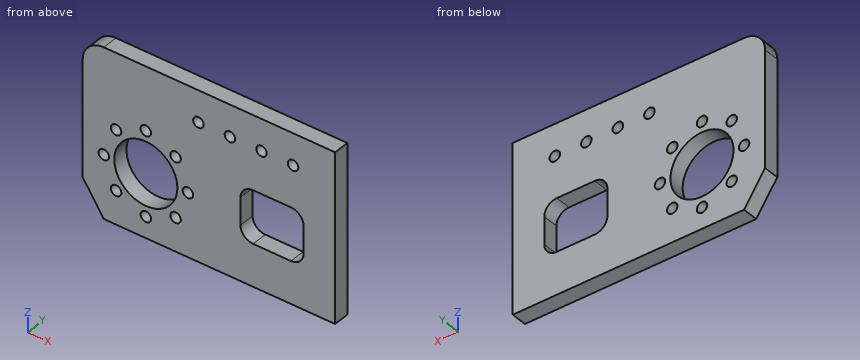
from build123d import *

# Parameters (mm, degrees)
SKETCH1_R           = 19.05
SKETCH1_R_2         = 3.175
BOSS_EXTRUDE1_DEPTH = 9.525


with BuildPart() as part:
    # Sketch1 → Boss-Extrude1 (new body)
    with BuildSketch(Plane(origin=(0, 0, 0), x_dir=(1, 0, 0), z_dir=(0, 1, 0))):
        with BuildLine():
            Line((0, -19.05), (12.7, 0))
            Line((12.7, 0), (152.4, 0))
            Line((152.4, 0), (152.4, -101.6))
            Line((152.4, -101.6), (12.7, -101.6))
            ThreePointArc((12.7, -101.6), (3.719743879, -97.880256121), (0, -88.9))
            Line((0, -88.9), (0, -19.05))
        make_face()
        with Locations((38.1, -38.1)):
            Circle(SKETCH1_R, mode=Mode.SUBTRACT)
        with Locations((56.060512242, -56.060512242)):
            Circle(SKETCH1_R_2, mode=Mode.SUBTRACT)
        with Locations((38.1, -63.5)):
            Circle(SKETCH1_R_2, mode=Mode.SUBTRACT)
        with Locations((20.139487758, -56.060512242)):
            Circle(SKETCH1_R_2, mode=Mode.SUBTRACT)
        with Locations((12.7, -38.1)):
            Circle(SKETCH1_R_2, mode=Mode.SUBTRACT)
        with Locations((20.139487758, -20.139487758)):
            Circle(SKETCH1_R_2, mode=Mode.SUBTRACT)
        with Locations((38.1, -12.7)):
            Circle(SKETCH1_R_2, mode=Mode.SUBTRACT)
        with Locations((56.060512242, -20.139487758)):
            Circle(SKETCH1_R_2, mode=Mode.SUBTRACT)
        with Locations((63.5, -38.1)):
            Circle(SKETCH1_R_2, mode=Mode.SUBTRACT)
        with Locations((69.85, -82.55)):
            Circle(SKETCH1_R_2, mode=Mode.SUBTRACT)
        with Locations((88.9, -82.55)):
            Circle(SKETCH1_R_2, mode=Mode.SUBTRACT)
        with Locations((107.95, -82.55)):
            Circle(SKETCH1_R_2, mode=Mode.SUBTRACT)
        with Locations((127, -82.55)):
            Circle(SKETCH1_R_2, mode=Mode.SUBTRACT)
        with BuildLine():
            Line((102.87, -25.4), (125.73, -25.4))
            ThreePointArc((125.73, -25.4), (131.118153673, -27.631846327), (133.35, -33.02))
            Line((133.35, -33.02), (133.35, -49.53))
            ThreePointArc((133.35, -49.53), (131.118153673, -54.918153673), (125.73, -57.15))
            Line((125.73, -57.15), (102.87, -57.15))
            ThreePointArc((102.87, -57.15), (97.481846327, -54.918153673), (95.25, -49.53))
            Line((95.25, -49.53), (95.25, -33.02))
            ThreePointArc((95.25, -33.02), (97.481846327, -27.631846327), (102.87, -25.4))
        make_face(mode=Mode.SUBTRACT)
    extrude(amount=BOSS_EXTRUDE1_DEPTH)


solid = part.part
Could you check a few things on this model? Use its own coordinates, in mm. Coordinates: 2 decimals unless noted, no trailing zeros. Order: outer loops, then holes, each group sorted by start corner. A loop starts at its lowest first (then second) coordinate and runs counter-clockwise, first axis right, second up. Notation, with made-up numbers: (-5.5, -24.75) -> (35.5, -24.75) arc R20 ccw to (35.5, 7.25) -> close; hole circle Ø1 at (-28, 50.5). An arc over 180 degrees is marked (long way). One line per item, written item: value. Start each with the question number.
1) Imagine slicing it at B-B on x = 114.5. List the corners of the cut face in (y, z) for me (3 decimals).
2) Imagine slicing it at C-C on x = 38.1. List the corners of the cut face in (y, z) for me (3 decimals).
3) Imagine slicing it at D-D on y = 2. Count the separate pieces of the cut face and the enclosed holes in it, plus the area to 3 significant figures.
4) Imagine slicing it at A-A on z = 38.1. List the corners of the cut face in (x, y) for me (3 decimals), plus the area to 3 significant figures.
5) I'm going to push a flat-ended pin straight in: pin 1 (5 mm diameter, centred on x = 127, z = 82.55, fed in from -Y). Where does the tip first touch, or does it pass through?
6) If I drill on L1, parallel to X at y = 3.25, z = 82.55 (3 decimals); L2, parallel to Z at x = 107.95, y = 4.75 (3 decimals); L3, parallel to Z at x = 38.1, y = 3.5 (3 decimals), over which ranges is the centre line in solid material (lowest first)? Write a range as [from, to].
Answer list:
1. outline: (0, 0) -> (9.525, 0) -> (9.525, 25.4) -> (0, 25.4) -> close; (0, 57.15) -> (9.525, 57.15) -> (9.525, 101.6) -> (0, 101.6) -> close
2. outline: (0, 0) -> (9.525, 0) -> (9.525, 9.525) -> (0, 9.525) -> close; (0, 15.875) -> (9.525, 15.875) -> (9.525, 19.05) -> (0, 19.05) -> close; (0, 57.15) -> (9.525, 57.15) -> (9.525, 60.325) -> (0, 60.325) -> close; (0, 66.675) -> (9.525, 66.675) -> (9.525, 101.6) -> (0, 101.6) -> close
3. separate pieces: 1
3. enclosed holes: 14
3. area: 12,600 mm2
4. outline: (0, 0) -> (9.525, 0) -> (9.525, 9.525) -> (0, 9.525) -> close; (15.875, 0) -> (19.05, 0) -> (19.05, 9.525) -> (15.875, 9.525) -> close; (57.15, 0) -> (60.325, 0) -> (60.325, 9.525) -> (57.15, 9.525) -> close; (66.675, 0) -> (95.25, 0) -> (95.25, 9.525) -> (66.675, 9.525) -> close; (133.35, 0) -> (152.4, 0) -> (152.4, 9.525) -> (133.35, 9.525) -> close
4. area: 605 mm2
5. pin 1: passes through
6. L1: x = [0, 66.675], [73.025, 85.725], [92.075, 104.775], [111.125, 123.825], [130.175, 152.4]
6. L2: z = [0, 25.4], [57.15, 79.375], [85.725, 101.6]
6. L3: z = [0, 9.525], [15.875, 19.05], [57.15, 60.325], [66.675, 101.6]
